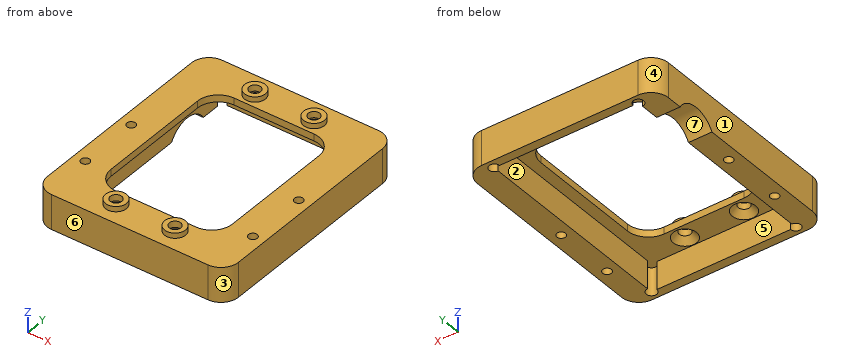
```python
from build123d import *

# Parameters (mm, degrees)
F0_W            = 55
F0_H            = 10
F1_DEPTH        = 32.5
F3_R            = 5
F4_DEPTH        = 12.5
F6_DEPTH        = 30
F7_DEPTH        = 3
F9_D            = 3.3
F9_CSINK_D      = 6.72
F9_CSINK_ANGLE  = 90
F10_R           = 3
F11_DEPTH       = 1.5
F12_D           = 3.3
F12_DEPTH       = 13.5
F12_CSINK_D     = 6.72
F12_CSINK_ANGLE = 90
F12_TIP         = 0.9914200214
F14_D           = 2.5
F14_DEPTH       = 13.5
F14_TIP         = 0.7510757738
F16_DEPTH       = 12


with BuildPart() as f1:
    # F0 (on Front) → F1 (new body, symmetric)
    with BuildSketch(Plane.XZ):
        Rectangle(F0_W, F0_H)
    extrude(amount=F1_DEPTH, both=True)

    # F3
    f3_edges = [f1.edges().sort_by_distance(p)[0] for p in [
        (27.5, -32.5, 0),
        (-27.5, -32.5, 0),
        (-27.5, 32.5, 0),
        (27.5, 32.5, 0),
    ]]
    fillet(f3_edges, radius=F3_R)

    # F2 (on Top) → F4 (cut, symmetric)
    with BuildSketch(Plane.XY):
        with BuildLine():
            Line((-11.5, -22.5), (11.5, -22.5))
            ThreePointArc((11.5, -22.5), (15.7426406871, -20.7426406871), (17.5, -16.5))
            Line((17.5, -16.5), (17.5, 16.5))
            ThreePointArc((17.5, 16.5), (15.7426406871, 20.7426406871), (11.5, 22.5))
            Line((11.5, 22.5), (-11.5, 22.5))
            ThreePointArc((-11.5, 22.5), (-15.7426406871, 20.7426406871), (-17.5, 16.5))
            Line((-17.5, 16.5), (-17.5, -16.5))
            ThreePointArc((-17.5, -16.5), (-15.7426406871, -20.7426406871), (-11.5, -22.5))
        make_face()
    extrude(amount=F4_DEPTH, both=True, mode=Mode.SUBTRACT)

    # F5 (on Top) → F6 (cut)
    with BuildSketch(Plane.XY):
        with BuildLine():
            ThreePointArc((-20.75, -28.5), (-21.8106601718, -31.0606601718), (-19.25, -30))
            Line((-19.25, -30), (-20.75, -30))
            Line((-20.75, -30), (-20.75, -28.5))
        make_face()
        with BuildLine():
            ThreePointArc((-20.75, -28.5), (-19.6893398282, -28.9393398282), (-19.25, -30))
            Line((-19.25, -30), (19.25, -30))
            ThreePointArc((19.25, -30), (19.6893398282, -28.9393398282), (20.75, -28.5))
            Line((20.75, -28.5), (20.75, 28.5))
            ThreePointArc((20.75, 28.5), (19.6893398282, 28.9393398282), (19.25, 30))
            Line((19.25, 30), (-19.25, 30))
            ThreePointArc((-19.25, 30), (-19.6893398282, 28.9393398282), (-20.75, 28.5))
            Line((-20.75, 28.5), (-20.75, -28.5))
        make_face()
        with BuildLine():
            Line((-20.75, -30), (-19.25, -30))
            ThreePointArc((-19.25, -30), (-19.6893398282, -28.9393398282), (-20.75, -28.5))
            Line((-20.75, -28.5), (-20.75, -30))
        make_face()
        with BuildLine():
            ThreePointArc((20.75, -28.5), (19.6893398282, -28.9393398282), (19.25, -30))
            Line((19.25, -30), (20.75, -30))
            Line((20.75, -30), (20.75, -28.5))
        make_face()
        with BuildLine():
            Line((20.75, -30), (19.25, -30))
            ThreePointArc((19.25, -30), (20.75, -31.5), (22.25, -30))
            ThreePointArc((22.25, -30), (21.8106601718, -28.9393398282), (20.75, -28.5))
            Line((20.75, -28.5), (20.75, -30))
        make_face()
        with BuildLine():
            ThreePointArc((-19.25, 30), (-21.8106601718, 31.0606601718), (-20.75, 28.5))
            Line((-20.75, 28.5), (-20.75, 30))
            Line((-20.75, 30), (-19.25, 30))
        make_face()
        with BuildLine():
            Line((-20.75, 30), (-20.75, 28.5))
            ThreePointArc((-20.75, 28.5), (-19.6893398282, 28.9393398282), (-19.25, 30))
            Line((-19.25, 30), (-20.75, 30))
        make_face()
        with BuildLine():
            ThreePointArc((19.25, 30), (19.6893398282, 28.9393398282), (20.75, 28.5))
            Line((20.75, 28.5), (20.75, 30))
            Line((20.75, 30), (19.25, 30))
        make_face()
        with BuildLine():
            Line((20.75, 30), (20.75, 28.5))
            ThreePointArc((20.75, 28.5), (21.8106601718, 28.9393398282), (22.25, 30))
            ThreePointArc((22.25, 30), (20.75, 31.5), (19.25, 30))
            Line((19.25, 30), (20.75, 30))
        make_face()
    extrude(amount=-F6_DEPTH, mode=Mode.SUBTRACT)

    # F5 (on Top) → F7 (cut)
    with BuildSketch(Plane.XY):
        with BuildLine():
            ThreePointArc((-20.75, -28.5), (-21.8106601718, -31.0606601718), (-19.25, -30))
            Line((-19.25, -30), (-20.75, -30))
            Line((-20.75, -30), (-20.75, -28.5))
        make_face()
        with BuildLine():
            ThreePointArc((-20.75, -28.5), (-19.6893398282, -28.9393398282), (-19.25, -30))
            Line((-19.25, -30), (19.25, -30))
            ThreePointArc((19.25, -30), (19.6893398282, -28.9393398282), (20.75, -28.5))
            Line((20.75, -28.5), (20.75, 28.5))
            ThreePointArc((20.75, 28.5), (19.6893398282, 28.9393398282), (19.25, 30))
            Line((19.25, 30), (-19.25, 30))
            ThreePointArc((-19.25, 30), (-19.6893398282, 28.9393398282), (-20.75, 28.5))
            Line((-20.75, 28.5), (-20.75, -28.5))
        make_face()
        with BuildLine():
            Line((-20.75, -30), (-19.25, -30))
            ThreePointArc((-19.25, -30), (-19.6893398282, -28.9393398282), (-20.75, -28.5))
            Line((-20.75, -28.5), (-20.75, -30))
        make_face()
        with BuildLine():
            ThreePointArc((20.75, -28.5), (19.6893398282, -28.9393398282), (19.25, -30))
            Line((19.25, -30), (20.75, -30))
            Line((20.75, -30), (20.75, -28.5))
        make_face()
        with BuildLine():
            Line((20.75, -30), (19.25, -30))
            ThreePointArc((19.25, -30), (20.75, -31.5), (22.25, -30))
            ThreePointArc((22.25, -30), (21.8106601718, -28.9393398282), (20.75, -28.5))
            Line((20.75, -28.5), (20.75, -30))
        make_face()
        with BuildLine():
            ThreePointArc((-19.25, 30), (-21.8106601718, 31.0606601718), (-20.75, 28.5))
            Line((-20.75, 28.5), (-20.75, 30))
            Line((-20.75, 30), (-19.25, 30))
        make_face()
        with BuildLine():
            Line((-20.75, 30), (-20.75, 28.5))
            ThreePointArc((-20.75, 28.5), (-19.6893398282, 28.9393398282), (-19.25, 30))
            Line((-19.25, 30), (-20.75, 30))
        make_face()
        with BuildLine():
            ThreePointArc((19.25, 30), (19.6893398282, 28.9393398282), (20.75, 28.5))
            Line((20.75, 28.5), (20.75, 30))
            Line((20.75, 30), (19.25, 30))
        make_face()
        with BuildLine():
            Line((20.75, 30), (20.75, 28.5))
            ThreePointArc((20.75, 28.5), (21.8106601718, 28.9393398282), (22.25, 30))
            ThreePointArc((22.25, 30), (20.75, 31.5), (19.25, 30))
            Line((19.25, 30), (20.75, 30))
        make_face()
    extrude(amount=F7_DEPTH, mode=Mode.SUBTRACT)

    # F9 (through all)
    with Locations(Plane(origin=(0, 0, 3), x_dir=(1, 0, 0), z_dir=(0, 0, -1))):
        with Locations((-8.5, -26.5042820722), (8.5, -26.5042820722)):
            CounterSinkHole(F9_D / 2, F9_CSINK_D / 2, counter_sink_angle=F9_CSINK_ANGLE)

    # F10 (on face) → F11 (join)
    with BuildSketch(Plane.XY.offset(5)):
        with Locations((8.5, 26.5042820722)):
            Circle(F10_R)
        with Locations((-8.5, 26.5042820722)):
            Circle(F10_R)
        with Locations((-8.5, -26.5)):
            Circle(F10_R)
        with Locations((8.5, -26.5)):
            Circle(F10_R)
    extrude(amount=F11_DEPTH)

    # F12
    with Locations(Plane(origin=(0, 0, 3), x_dir=(1, 0, 0), z_dir=(0, 0, -1))):
        with Locations((-8.5, -26.5042820722), (8.5, -26.5042820722), (8.5, 26.5), (-8.5, 26.5)):
            CounterSinkHole(F12_D / 2, F12_CSINK_D / 2, depth=F12_DEPTH, counter_sink_angle=F12_CSINK_ANGLE)
            with Locations((0, 0, -(F12_DEPTH + F12_TIP / 2))):  # 118° drill point
                Cone(0, F12_D / 2, F12_TIP, mode=Mode.SUBTRACT)

    # F14
    with Locations(Plane(origin=(0, 0, -5), x_dir=(1, 0, 0), z_dir=(0, 0, -1))):
        with Locations((-24.125, 0), (24.125, 0), (-24.125, 17.5), (24.125, 17.5)):
            Hole(F14_D / 2, depth=F14_DEPTH)
            with Locations((0, 0, -(F14_DEPTH + F14_TIP / 2))):  # 118° drill point
                Cone(0, F14_D / 2, F14_TIP, mode=Mode.SUBTRACT)

    # F15 (on face) → F16 (cut)
    with BuildSketch(Plane(origin=(-27.5, 0, 0), x_dir=(0, -1, 0), z_dir=(-1, 0, 0))):
        with BuildLine():
            Line((-23.0304132, -5), (-10.906057547, -5))
            ThreePointArc((-10.906057547, -5), (-16.9682353735, -1.5), (-23.0304132, -5))
        make_face()
    extrude(amount=-F16_DEPTH, mode=Mode.SUBTRACT)


solid = f1.part
```
Here's how the part is built. I have some questions about the finished solid (model axes, mm). Face numbers are marked on the shaded views. A direction names the side the tool comes from. Round coordinates to 2 decimals unless told otherwise and drop trailing zeros. Loops run counter-clockwise (first coordinate to the right, second up) from the corner with the lowest first, then second, coordinate; pieces in that order, holes last.
1. If I drill on probe 1 along X at (y, z) = (-17.5, -0.75) (3 decimals); probe 2 along Y at (x, z) = (-8.5, 5.5); probe 3 along X at (y, z) = (-12, 2.5), over which ranges is the centre line in solid material (lowest first)?
Answers:
probe 1: x = -27.5 to -25.375, -22.875 to -20.75, 20.75 to 22.875, 25.375 to 27.5
probe 2: y = -29.5 to -28.15, -24.85 to -23.5, 23.5 to 24.85, 28.15 to 29.5
probe 3: x = -27.5 to -20.75, 20.75 to 27.5
2. Suppose I cut it at A-A, the plane y = -26.5. Please give me the cut outline in (x, z), and give its area (3 significant figures).
Answers:
outline: (-27.5, -5) - (-20.75, -5) - (-20.75, 3) - (-11.86, 3) - (-10.15, 4.71) - (-10.15, 6.5) - (-11.5, 6.5) - (-11.5, 5) - (-27.5, 5) - close; (-6.85, 4.71) - (-5.14, 3) - (5.14, 3) - (6.85, 4.71) - (6.85, 6.5) - (5.5, 6.5) - (5.5, 5) - (-5.5, 5) - (-5.5, 6.5) - (-6.85, 6.5) - close; (10.15, 4.71) - (11.86, 3) - (20.75, 3) - (20.75, -5) - (27.5, -5) - (27.5, 5) - (11.5, 5) - (11.5, 6.5) - (10.15, 6.5) - close
area: 207 mm2
3. For the marked faces 5, 6 and 7, which set-ups out of +Z, -Z, +X, -X, +Y, -Y let a thin tool reach every point of the face, with its end or its side?
Answers:
face 5: -Z
face 6: +Z, -Z, +X, -X, -Y
face 7: -Z, -X
4. Thinking about a two-plate mould opening in Y: for the marked faces 1, 2, 3 and 4, which applies, released by +Y, released by -Y, zero draft, split by the parting line, or undercut?
Answers:
face 1: zero draft
face 2: undercut
face 3: released by -Y
face 4: released by +Y
5. Suppose I cut it at D-D, the plane y = 0. Please give me the cut outline in (x, z) (3 decimals).
Answers:
outline: (-27.5, -5) - (-25.375, -5) - (-25.375, 5) - (-27.5, 5) - close; (-22.875, -5) - (-20.75, -5) - (-20.75, 3) - (-17.5, 3) - (-17.5, 5) - (-22.875, 5) - close; (17.5, 3) - (20.75, 3) - (20.75, -5) - (22.875, -5) - (22.875, 5) - (17.5, 5) - close; (25.375, -5) - (27.5, -5) - (27.5, 5) - (25.375, 5) - close
6. Suppose I cut it at B-B, the plane x = -8.5. Give the number of separate pieces and of enclosed holes in the cut face, and give its area (3 significant figures).
Answers:
separate pieces: 4
enclosed holes: 0
area: 69.1 mm2
7. Will these pins go through, and if not, where does the flat tip stop? pin 1 (3 mm diameter, centred on x = -24.125, y = 0, fed in from -Z); pin 2 (3 mm diameter, centred on x = 8.5, y = -26.5, fed in from -Z); pin 3 (4.5 mm diameter, centred on x = -8.5, y = -26.5, fed in from -Z); pin 4 (8 mm diameter, centred on x = -15, y = -21, fed in from -Z).
Answers:
pin 1: stops at z = -5
pin 2: passes through
pin 3: stops at z = 4.11
pin 4: stops at z = 3
8. Suppose I cut it at C-C, the plane z = 5.75. Please give me the cut outline in (x, y).
Answers:
outline: circle Ø6 at (-8.5, -26.5); circle Ø6 at (-8.5, 26.5); circle Ø6 at (8.5, -26.5); circle Ø6 at (8.5, 26.5); hole circle Ø3.3 at (-8.5, -26.5); hole circle Ø3.3 at (-8.5, 26.5); hole circle Ø3.3 at (8.5, -26.5); hole circle Ø3.3 at (8.5, 26.5)
